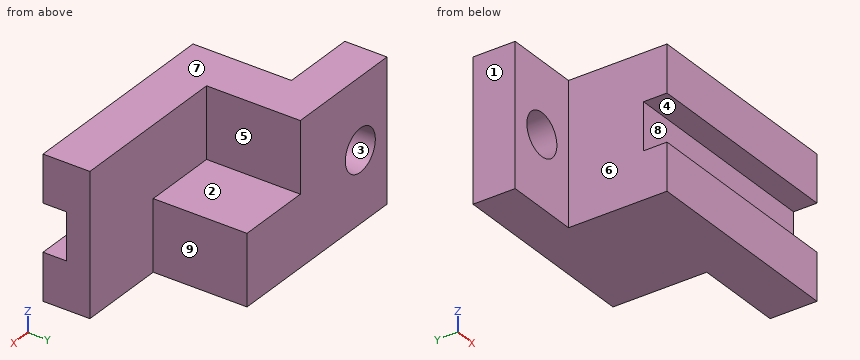
Autodesk Fusion 360 part; units mm, degrees
sketch "Sketch1" plane through (0, 0, 0) normal (0, 1, 0) x (1, 0, 0)
  line L0 (0, 0) -> (61, 0)
  line L1 (61, 0) -> (61, -30)
  line L2 (61, -30) -> (0, -30)
  line L3 (0, -30) -> (0, 0)
  dimension "d1" = 61
  dimension "d2" = 30
extrude "Extrude1" add sketch "Sketch1" along normal blind 10
sketch "Sketch2" plane through (0, 10, 0) normal (0, 1, 0) x (-1, 0, 0)
  line L0 (0, 30) -> (-61, 30)
  line L1 (-61, 30) -> (-61, 0)
  line L2 (-61, 0) -> (0, 0)
  line L3 (0, 0) -> (0, 30)
  line L4 (0, 0) -> (-26, 0)
  line L5 (-26, 0) -> (-26, 30)
  line L6 (-26, 30) -> (0, 30)
  line L7 (0, 30) -> (0, 0)
  dimension "d5" = 26
extrude "Extrude2" add sketch "Sketch2" along normal blind 20 contours L0 L2 L3 L4 L5 L6 L7
sketch "Sketch3" plane through (0, 30, 0) normal (0, 1, 0) x (-1, 0, 0)
  line L0 (0, 30) -> (-26, 30)
  line L1 (-26, 30) -> (-26, 0)
  line L2 (-26, 0) -> (0, 0)
  line L3 (0, 0) -> (0, 30)
  line L4 (-26, 0) -> (-42, 0)
  line L5 (-42, 0) -> (-42, 15)
  line L6 (-42, 15) -> (-26, 15)
  line L7 (-26, 15) -> (-26, 0)
  dimension "d8" = 16
  dimension "d9" = 15
extrude "Extrude3" add sketch "Sketch3" against normal up to surface (20 mm away) contours L1 L4 L5 L6 L7
sketch "Sketch4" plane through (0, 0, 30) normal (0, 0, 1) x (1, 0, 0)
  line L0 (0, 0) -> (61, 0)
  line L1 (61, 0) -> (61, 10)
  line L2 (61, 10) -> (26, 10)
  line L3 (26, 10) -> (26, 30)
  line L4 (26, 30) -> (0, 30)
  line L5 (0, 30) -> (0, 0)
  line L6 (0, 0) -> (16, 0)
  line L7 (16, 0) -> (16, 21)
  line L8 (16, 21) -> (0, 21)
  line L9 (0, 21) -> (0, 0)
  dimension "d12" = 16
  dimension "d13" = 21
extrude "Extrude4" cut sketch "Sketch4" against normal blind 30 contours L0 L5 L6 L7 L8 L9
sketch "Sketch5" plane through (0, 30, 0) normal (0, 1, 0) x (-1, 0, 0)
  line L0 (0, 30) -> (-26, 30)
  line L1 (-26, 30) -> (-26, 15)
  line L2 (-26, 15) -> (-42, 15)
  line L3 (-42, 15) -> (-42, 0)
  line L4 (-42, 0) -> (0, 0)
  line L5 (0, 0) -> (0, 30)
  line L6 (28.1028, 15) -> (-28.1028, 15) construction
  circle A0 centre (-8, 15) radius 4.5
  dimension "d16" = 9
  dimension "d17" = 8
extrude "Extrude5" cut sketch "Sketch5" against normal blind 9 contours A0
sketch "Sketch6" plane through (61, 0, 0) normal (1, 0, 0) x (0, 0, -1)
  line L0 (-30, 0) -> (0, 0)
  line L1 (0, 0) -> (0, 10)
  line L2 (0, 10) -> (-30, 10)
  line L3 (-30, 10) -> (-30, 0)
  line L4 (-20, 0) -> (-20, 5)
  line L5 (-20, 5) -> (-10, 5)
  line L6 (-10, 5) -> (-10, 0)
  dimension "d20" = 10
  dimension "d21" = 5
  dimension "d22" = 5
  dimension "d23" = 10
extrude "Extrude6" cut sketch "Sketch6" against normal blind 45 contours L0 L4 L5 L6
Geometry check sheet. Reference: the model listing, model coordinates, mm. Face numbers are marked on the shaded views. A direction names the side the tool comes from. Coordinates: 2 decimals unless noted, no trailing zeros. Order: outer loops, then holes, each group sorted by start corner. A loop starts at its lowest first (then second) coordinate and runs counter-clockwise, first axis right, second up. Notation, with made-up numbers: (67, -38) - (89, -38) arc R23 ccw to (89, -6) - close; hole circle Ø6 at (13, 29). An arc over 180 degrees is marked (long way). Answer in a Markdown table with one row per item. Add a question column.
1) Gauge pin test, flat ends, axial feed: P1, Ø6, axis at y = 16.5, z = 12.5, coming from the +X side; P2, Ø5, axis at x = 10, z = 14.5, coming from the -Y side; P3, Ø5, axis at x = 30, y = 23.5, coming from the +Z side. Record the tip position at first contact, or that the pin passes through.
2) Cross-section at C-C, the plane x = 27. Record the cut outline in (y, z), then the cut area to 3 significant figures.
3) Cross-section at A-A, the plane x = 8. Record the cut outline in (y, z).
4) Cross-section at D-D, the plane z = 21.75. Record the cut outline in (x, y), then the cut area to 3 significant figures.
5) Release check for a two-part mould opening along Z. For the marked faces 1, 2, 3 and 4 record: +Z half, -Z half, draft (parallel to the pull), parting line (faces both ways), or undercut.
6) Set-up check for the marked faces 5, 6, 7, 8 and 9: record each of +Z, -Z, +X, -X, +Y, -Y from which the full face is reachable in a straight line by a thin tool's end or side.
7) Cross-section at B-B, the plane y = 26.5. Record the cut outline in (x, z).
8) Material ranges on line 1 along Z through (x, y) = (8, 27.75); line 2 along Y through (x, z) = (31, 10.5); line 3 along X through (y, z) = (14.5, 10.5), recorded low to high. Write a range as [from, to].
Check result:
| question | item | result |
|---|---|---|
| 1 | P1 | stops at x = 42 |
| 1 | P2 | stops at y = 21 |
| 1 | P3 | stops at z = 15 |
| 2 | outline | (0, 0) - (30, 0) - (30, 15) - (10, 15) - (10, 30) - (0, 30) - (0, 20) - (5, 20) - (5, 10) - (0, 10) - close |
| 2 | area | 550 mm² |
| 3 | outline | (21, 0) - (30, 0) - (30, 10.5) - (21, 10.5) - close; (21, 19.5) - (30, 19.5) - (30, 30) - (21, 30) - close |
| 4 | outline | (0, 21) - (16, 21) - (16, 0) - (61, 0) - (61, 10) - (26, 10) - (26, 30) - (0, 30) - close |
| 4 | area | 794 mm² |
| 5 | face 1 | draft |
| 5 | face 2 | +Z half |
| 5 | face 3 | undercut |
| 5 | face 4 | undercut |
| 6 | face 5 | +Z, +X, +Y |
| 6 | face 6 | +Z, -Z, -X, -Y |
| 6 | face 7 | +Z, +X, -X, +Y, -Y |
| 6 | face 8 | +X, -X, -Y |
| 6 | face 9 | +Z, -Z, +X, +Y |
| 7 | outline | (0, 0) - (42, 0) - (42, 15) - (26, 15) - (26, 30) - (0, 30) - close; hole circle Ø9 at (8, 15) |
| 8 | line 1 | z = [0, 10.5], [19.5, 30] |
| 8 | line 2 | y = [5, 30] |
| 8 | line 3 | x = [16, 42] |
